Autodesk Inventor part; units mm, degrees
ref_plane "YZ Plane" through (0, 0, 0) normal (1, 0, 0) x (0, 1, 0)
ref_plane "XZ Plane" through (0, 0, 0) normal (0, 1, 0) x (-1, 0, 0)
ref_plane "XY Plane" through (0, 0, 0) normal (0, 0, 1) x (1, 0, 0)
sketch "Sketch2" plane through (0, 0, 0) normal (0, 1, 0) x (-1, 0, 0)
  line L0 (127, 0) -> (177.8, 0)
  line L1 (177.8, 0) -> (177.8, -203.2)
  line L2 (177.8, -203.2) -> (0, -203.2)
  line L3 (0, -203.2) -> (0, -114.3)
  line L4 (0, -114.3) -> (127, -114.3)
  line L5 (127, -114.3) -> (127, 0)
  point P0 (0, 0)
  dimension "d0" = 203.2
  dimension "d1" = 177.8
  dimension "d65" = 50.8
  dimension "d66" = 88.9
extrude "Extrusion1" add sketch "Sketch2" along normal blind 12.7
sketch "Sketch3" plane through (0, 12.7, 0) normal (0, 1, 0) x (1, 0, 0)
  line L0 (-127, 0) -> (-177.8, 0)
  line L1 (-177.8, 0) -> (-177.8, 203.2)
  line L2 (-177.8, 203.2) -> (0, 203.2)
  line L3 (0, 203.2) -> (0, 114.3)
  line L4 (-171.45, 196.85) -> (-171.45, 6.35)
  line L5 (-171.45, 6.35) -> (-133.35, 6.35)
  line L6 (-6.35, 120.65) -> (-6.35, 196.85)
  line L7 (-6.35, 196.85) -> (-171.45, 196.85)
  line L8 (0, 114.3) -> (-127, 114.3)
  line L9 (-127, 114.3) -> (-127, 0)
  line L10 (-6.35, 120.65) -> (-133.35, 120.65)
  line L11 (-133.35, 120.65) -> (-133.35, 6.35)
  line L12 (-127, 0) -> (-127, 114.3)
  line L13 (0, 114.3) -> (0, 203.2)
  point P0 (0, 0)
  point P1 (-127, 6.35)
  point P2 (0, 120.65)
  point P3 (-114.3, 0)
  point P4 (-6.35, 114.3)
  dimension "d4" = 6.35
  dimension "d61" = 120.65
  dimension "d62" = 107.95
  dimension "d63" = 6.35
  dimension "d64" = 6.35
  dimension "d76" = 0
  dimension "d77" = 6.35
  dimension "d78" = 0
extrude "Extrusion2" add sketch "Sketch3" along normal blind 114.3
sketch "Sketch5" plane through (0, 12.7, 0) normal (0, 1, 0) x (1, 0, 0)
  line L0 (-114.3, 114.3) -> (-114.3, 6.35)
  line L1 (-6.35, 120.65) -> (-6.3512, 120.1928)
  line L2 (-171.45, 114.3) -> (-114.3, 114.3)
  line L3 (-171.45, 6.35) -> (-171.45, 196.85)
  line L4 (-133.35, 6.35) -> (-171.45, 6.35)
  line L5 (-171.45, 120.65) -> (-57.15, 120.65)
  line L6 (-107.95, 114.3) -> (-107.95, 6.35)
  line L7 (-171.45, 120.65) -> (-6.35, 120.65)
  line L8 (-107.95, 114.3) -> (-6.35, 114.3)
  line L9 (-6.35, 196.85) -> (-6.35, 120.65)
  line L10 (-171.45, 120.65) -> (-171.45, 114.3)
  line L11 (-6.35, 120.65) -> (-6.35, 114.3)
  line L12 (-6.35, 120.65) -> (-6.35, 114.3)
  line L13 (-133.35, 6.35) -> (-107.95, 6.35)
  line L14 (-171.45, 6.35) -> (-133.35, 6.35)
  point P0 (-6.35, 6.35)
  dimension "d37" = 107.95
  dimension "d38" = 6.35
  dimension "d58" = 101.6
  dimension "d60" = 6.35
extrude "Extrusion5" [suppressed]
sketch "Sketch6" plane through (0, 0, 0) normal (0, -1, 0) x (1, 0, 0)
  line L0 (0, -203.2) -> (-177.8, 0) construction
  circle A0 centre (-88.9, -101.6) radius 101.6 construction
  line L1 (-177.8, -203.2) -> (0, 0) construction
  point P0 (-155.8041, -178.0618)
  point P1 (-155.8041, -25.1382)
  point P2 (-21.9959, -25.1382)
  point P3 (-21.9959, -178.0618)
  dimension "d25" = 203.2
hole "Hole1" [suppressed]
sketch "Sketch7" plane through (-6.35, 12.7, -196.85) normal (-1, 0, 0) x (0, 0, 1)
  line L0 (76.2, 0) -> (0, 0)
  line L1 (76.2, 114.3) -> (76.2, 0)
  line L2 (0, 0) -> (76.2, 0)
  line L3 (76.2, 0) -> (76.2, 63.5)
  line L4 (76.2, 63.5) -> (0, 63.5)
  line L5 (0, 63.5) -> (0, 0)
  point P0 (196.85, -12.7)
  dimension "d39" = 63.5
extrude "Extrusion6" [suppressed]
sketch "Sketch10" plane through (0, 12.7, 0) normal (0, 1, 0) x (1, 0, 0)
  line L0 (-164.5, 98.825) -> (-135.392, 98.825) construction
  line L1 (-135.392, 98.825) -> (-135.392, 21.825) construction
  line L2 (-135.392, 21.825) -> (-164.5, 21.825) construction
  line L3 (-164.5, 21.825) -> (-164.5, 98.825) construction
  line L4 (-171.45, 6.35) -> (-171.45, 196.85)
  line L5 (-133.35, 114.3) -> (-171.45, 114.3)
  line L6 (-171.45, 6.35) -> (-133.35, 6.35)
  circle A0 centre (-135.392, 98.825) radius 1.6
  circle A1 centre (-164.5, 98.825) radius 1.6
  circle A2 centre (-135.392, 21.825) radius 1.6
  circle A3 centre (-164.5, 21.825) radius 1.6
  point P0 (0, 0)
  point P1 (-127, 114.3)
  point P2 (-127, 6.35)
  dimension "d40" = 6.95
  dimension "d41" = 29.108
  dimension "d42" = 77
  dimension "d43" = 15.475
  dimension "d44" = 15.475
  dimension "d45" = 3.2
  dimension "d46" = 3.2
  dimension "d47" = 3.2
  dimension "d48" = 3.2
extrude "Extrusion7" cut sketch "Sketch10" against normal through all
sketch "Sketch11" plane through (-177.8, 0, -203.2) normal (-1, 0, 0) x (0, 0, 1)
  line L0 (203.2, 0) -> (203.2, 127)
  line L1 (203.2, 20.5386) -> (0, 20.5386) construction
  line L2 (0, 0) -> (0, 127)
  line L3 (196.85, 127) -> (6.35, 127)
  circle A0 centre (142.875, 67.55) radius 10
  line L4 (0, 0) -> (203.2, 0)
  point P0 (88.9, 127)
  dimension "d51" = 20
  dimension "d52" = 67.55
  dimension "d53" = 53.975
  dimension "d54" = 53.975
extrude "Extrusion8" cut sketch "Sketch11" against normal up to surface (6.35 mm away)
sketch "Sketch14" plane through (0, 127, 0) normal (0, 1, 0) x (1, 0, 0)
  line L0 (-177.8, 0) -> (-127, 0)
  line L1 (-127, 0) -> (-120.65, 0)
  line L2 (-120.65, 0) -> (-120.65, 6.35)
  line L3 (-120.65, 6.35) -> (-127, 6.35)
  line L4 (-127, 6.35) -> (-127, 0)
  line L5 (-177.8, 0) -> (-171.45, 0)
  line L6 (-171.45, 0) -> (-171.45, -6.35)
  line L7 (-171.45, -6.35) -> (-177.8, -6.35)
  line L8 (-177.8, -6.35) -> (-177.8, 0)
  point P0 (0, 0)
  dimension "d79" = 6.35
  dimension "d80" = 6.35
  dimension "d81" = 6.35
  dimension "d82" = 6.35
extrude "Extrusion11" add sketch "Sketch14" against normal up to surface (114.3 mm away)
sketch "Sketch15" plane through (0, 127, 0) normal (0, 1, 0) x (1, 0, 0)
  circle A0 centre (-135.392, 21.825) radius 1.6
  circle A1 centre (-135.392, 98.825) radius 1.6
  circle A2 centre (-164.5, 98.825) radius 1.6
  circle A3 centre (-164.5, 21.825) radius 1.6
  line L0 (-6.35, 196.85) -> (-171.45, 196.85)
  line L1 (-171.45, 196.85) -> (-171.45, 6.35)
  line L2 (-171.45, 6.35) -> (-133.35, 6.35)
  line L3 (-133.35, 6.35) -> (-133.35, 120.65)
  line L4 (-133.35, 120.65) -> (-6.35, 120.65)
  line L5 (-6.35, 120.65) -> (-6.35, 196.85)
  line L6 (-133.35, 120.65) -> (-127, 120.65)
  line L7 (-127, 120.65) -> (-127, 127)
  line L8 (-127, 127) -> (-133.35, 127)
  line L9 (-133.35, 127) -> (-133.35, 120.65)
  line L10 (-171.45, 196.85) -> (-6.35, 196.85)
  line L11 (-6.35, 196.85) -> (-6.35, 120.65)
  line L12 (-6.35, 120.65) -> (-133.35, 120.65)
  line L13 (-133.35, 120.65) -> (-133.35, 6.35)
  line L14 (-133.35, 6.35) -> (-171.45, 6.35)
  line L15 (-171.45, 6.35) -> (-171.45, 196.85)
  line L16 (-177.8, 203.2) -> (-177.8, -6.35)
  line L17 (-177.8, -6.35) -> (-171.45, -6.35)
  line L18 (-171.45, -6.35) -> (-171.45, 0)
  line L19 (-171.45, 0) -> (-120.65, 0)
  line L20 (-120.65, 0) -> (-120.65, 6.35)
  line L21 (-120.65, 6.35) -> (-127, 6.35)
  line L22 (-127, 6.35) -> (-127, 114.3)
  line L23 (-127, 114.3) -> (0, 114.3)
  line L24 (0, 114.3) -> (0, 203.2)
  line L25 (0, 203.2) -> (-177.8, 203.2)
  line L26 (0, 114.3) -> (6.35, 114.3)
  line L27 (6.35, 114.3) -> (6.35, 120.65)
  line L28 (6.35, 120.65) -> (0, 120.65)
  line L29 (0, 120.65) -> (0, 114.3)
  line L30 (0, 114.3) -> (0, 203.2)
  line L31 (0, 203.2) -> (-6.35, 203.2)
  line L32 (-6.35, 203.2) -> (-6.35, 209.55)
  line L33 (-6.35, 209.55) -> (0, 209.55)
  line L34 (0, 209.55) -> (0, 203.2)
  line L35 (0, 203.2) -> (-177.8, 203.2)
  line L36 (-177.8, 203.2) -> (-184.15, 203.2)
  line L37 (-184.15, 203.2) -> (-184.15, 196.85)
  line L38 (-184.15, 196.85) -> (-177.8, 196.85)
  line L39 (-177.8, 196.85) -> (-177.8, 203.2)
  point P0 (0, 0)
  dimension "d85" = 6.35
  dimension "d86" = 6.35
  dimension "d87" = 6.35
  dimension "d88" = 6.35
  dimension "d89" = 6.35
  dimension "d90" = 6.35
  dimension "d91" = 6.35
extrude "Extrusion12" add sketch "Sketch15" against normal up to surface (114.3 mm away) contours L4 L9 L8 L7 | L16 L38 L37 L36 | L32 L33 L34 L25 | L28 L27 L26 L24
equation "\"d43\" = d44"
properties part number "RSX Structure" material "Aluminum 6061"
Geometry check sheet. Reference: the model listing, model coordinates, mm. A direction names the side the tool comes from. Coordinates: 2 decimals unless noted, no trailing zeros. Order: outer loops, then holes, each group sorted by start corner. A loop starts at its lowest first (then second) coordinate and runs counter-clockwise, first axis right, second up. Notation, with made-up numbers: (24.25, -39.5) - (76.25, -39.5) arc R31 cw to (76.25, -8.5) - close; hole circle Ø4 at (54.25, 76). An arc over 180 degrees is marked (long way). Answer as a JSON object with one key per item and string values. Group by question number.
Item 1: Depth check by flat-ended pin: pin 1 Ø1 at (x, z) = (-13.5, -142.5) entering from +Y; pin 2 Ø12 at (x, y) = (-90, 42.5) entering from -Z; pin 3 Ø17 at (x, y) = (-148.5, 54) entering from +Z; pin 4 Ø4 at (x, z) = (-164.5, -21.825) entering from -Y. Enter the tip coordinate at first touch or a pass-through.
Item 2: Sectioned sample at A-A, the plane z = -181.5. Record the cut outline in (x, y), and give its area (3 significant figures).
Item 3: Sectioned sample at D-D, the plane z = -58.5. Record the cut outline in (x, y), and give its area (3 significant figures).
Item 4: Scan lines: probe 1 along X at (y, z) = (50.5, -166); probe 2 along X at (y, z) = (41.5, -62.5); probe 3 along X at (y, z) = (53.5, -122). Record each from-to range of solid material in increasing order.
Item 5: Draft check along Z on faces 1 (the face through (-88, 69, -196.85)), 2 (the face through (-181, 71, -196.85)), 3 (the face through (-171.45, 71, 3)). Enter one of: +Z half, -Z half, draft (parallel to the pull), parting line (faces both ways), or undercut.
Item 6: Sectioned sample at C-C, the plane x = -37.5. Record the cut outline in (y, z).
Item 7: Sectioned sample at B-B, the plane y = 82. Record the cut outline in (x, z).
Item 8: Tool access check on faces 4 (the face through (-6.35, 71, -206)), 5 (the face through (-124, 71, -6.35)), 6 (the face through (-120.65, 71, -3)), 7 (the face through (-130, 71, -127)), 8 (the face through (3, 71, -120.65)). Record the directions out of +Z, -Z, +X, -X, +Y, -Y that give a thin tool (end or side, any length) a straight path to the whole face; none if there is none.
Resolved:
{
 "1": {"pin 1": "y = 12.7", "pin 2": "z = -203.2", "pin 3": "z = 0", "pin 4": "y = 0"},
 "2": {"outline": "(-177.8, 0) - (0, 0) - (0, 127) - (-6.35, 127) - (-6.35, 12.7) - (-171.45, 12.7) - (-171.45, 127) - (-177.8, 127) - close", "area": "3,710 mm^2"},
 "3": {"outline": "(-177.8, 0) - (-127, 0) - (-127, 127) - (-133.35, 127) - (-133.35, 12.7) - (-171.45, 12.7) - (-171.45, 57.72) - (-177.8, 57.72) - close; (-177.8, 77.38) - (-171.45, 77.38) - (-171.45, 127) - (-177.8, 127) - close", "area": "1,970 mm^2"},
 "4": {"probe 1": "-177.8 to -171.45, -6.35 to 0", "probe 2": "-177.8 to -171.45, -133.35 to -127", "probe 3": "-177.8 to -171.45, -133.35 to -127, -6.35 to 0"},
 "5": {"face 1": "undercut", "face 2": "+Z half", "face 3": "draft"},
 "6": {"outline": "(0, -203.2) - (127, -203.2) - (127, -196.85) - (12.7, -196.85) - (12.7, -120.65) - (127, -120.65) - (127, -114.3) - (0, -114.3) - close"},
 "7": {"outline": "(-184.15, -203.2) - (-6.35, -203.2) - (-6.35, -209.55) - (0, -209.55) - (0, -120.65) - (6.35, -120.65) - (6.35, -114.3) - (-127, -114.3) - (-127, -6.35) - (-120.65, -6.35) - (-120.65, 0) - (-171.45, 0) - (-171.45, 6.35) - (-177.8, 6.35) - (-177.8, -196.85) - (-184.15, -196.85) - close; hole (-171.45, -196.85) - (-6.35, -196.85) - (-6.35, -120.65) - (-127, -120.65) - (-127, -127) - (-133.35, -127) - (-133.35, -6.35) - (-171.45, -6.35) - close"},
 "8": {"face 4": "-Z, -X, +Y, -Y", "face 5": "+X, +Y, -Y", "face 6": "+Z, +X, +Y, -Y", "face 7": "+Y", "face 8": "-Z, +X, +Y, -Y"}
}
